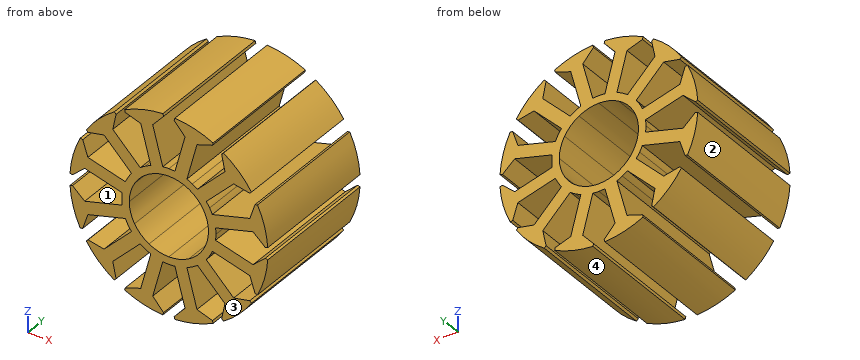
```python
from build123d import *

# Parameters (mm, degrees)
BOSS_EXTRUDE1_DEPTH = 27


with BuildPart() as part:
    # Sketch1 → Boss-Extrude1 (new body)
    with BuildSketch(Plane(origin=(0, 0, 0), x_dir=(1, 0, 0), z_dir=(0, 1, 0))):
        with BuildLine():
            Line((1.229996254, 9.420037644), (3.261041046, 17))
            Line((3.261041046, 17), (1.075459685, 19.463398226))
            Line((1.075459685, 19.463398226), (1.209434281, 19.963398226))
            ThreePointArc((1.209434281, 19.963398226), (5.176380902, 19.318516526), (8.934298302, 17.89352715))
            Line((8.934298302, 17.89352715), (8.800323705, 17.39352715))
            Line((8.800323705, 17.39352715), (5.675855612, 16.352952387))
            Line((5.675855612, 16.352952387), (3.64481082, 8.772990031))
            ThreePointArc((3.64481082, 8.772990031), (4.206265872, 8.5180589), (4.75, 8.227241336))
            ThreePointArc((4.75, 8.227241336), (5.273722462, 7.90176255), (5.775226824, 7.542993777))
            Line((5.775226824, 7.542993777), (11.324144388, 13.091911341))
            Line((11.324144388, 13.091911341), (10.66307452, 16.318067465))
            Line((10.66307452, 16.318067465), (11.029099924, 16.684092869))
            ThreePointArc((11.029099924, 16.684092869), (14.142135624, 14.142135624), (16.684092869, 11.029099924))
            Line((16.684092869, 11.029099924), (16.318067465, 10.66307452))
            Line((16.318067465, 10.66307452), (13.091911341, 11.324144388))
            Line((13.091911341, 11.324144388), (7.542993777, 5.775226824))
            ThreePointArc((7.542993777, 5.775226824), (7.90176255, 5.273722462), (8.227241336, 4.75))
            ThreePointArc((8.227241336, 4.75), (8.5180589, 4.206265872), (8.772990031, 3.64481082))
            Line((8.772990031, 3.64481082), (16.352952387, 5.675855612))
            Line((16.352952387, 5.675855612), (17.39352715, 8.800323705))
            Line((17.39352715, 8.800323705), (17.89352715, 8.934298302))
            ThreePointArc((17.89352715, 8.934298302), (19.318516526, 5.176380902), (19.963398226, 1.209434281))
            Line((19.963398226, 1.209434281), (19.463398226, 1.075459685))
            Line((19.463398226, 1.075459685), (17, 3.261041046))
            Line((17, 3.261041046), (9.420037644, 1.229996254))
            ThreePointArc((9.420037644, 1.229996254), (9.479988334, 0.61629635), (9.5, 0))
            ThreePointArc((9.5, 0), (9.479988334, -0.61629635), (9.420037644, -1.229996254))
            Line((9.420037644, -1.229996254), (17, -3.261041046))
            Line((17, -3.261041046), (19.463398226, -1.075459685))
            Line((19.463398226, -1.075459685), (19.963398226, -1.209434281))
            ThreePointArc((19.963398226, -1.209434281), (19.318516526, -5.176380902), (17.89352715, -8.934298302))
            Line((17.89352715, -8.934298302), (17.39352715, -8.800323705))
            Line((17.39352715, -8.800323705), (16.352952387, -5.675855612))
            Line((16.352952387, -5.675855612), (8.772990031, -3.64481082))
            ThreePointArc((8.772990031, -3.64481082), (8.5180589, -4.206265872), (8.227241336, -4.75))
            ThreePointArc((8.227241336, -4.75), (7.90176255, -5.273722462), (7.542993777, -5.775226824))
            Line((7.542993777, -5.775226824), (13.091911341, -11.324144388))
            Line((13.091911341, -11.324144388), (16.318067465, -10.66307452))
            Line((16.318067465, -10.66307452), (16.684092869, -11.029099924))
            ThreePointArc((16.684092869, -11.029099924), (14.142135624, -14.142135624), (11.029099924, -16.684092869))
            Line((11.029099924, -16.684092869), (10.66307452, -16.318067465))
            Line((10.66307452, -16.318067465), (11.324144388, -13.091911341))
            Line((11.324144388, -13.091911341), (5.775226824, -7.542993777))
            ThreePointArc((5.775226824, -7.542993777), (5.273722462, -7.90176255), (4.75, -8.227241336))
            ThreePointArc((4.75, -8.227241336), (4.206265872, -8.5180589), (3.64481082, -8.772990031))
            Line((3.64481082, -8.772990031), (5.675855612, -16.352952387))
            Line((5.675855612, -16.352952387), (8.800323705, -17.39352715))
            Line((8.800323705, -17.39352715), (8.934298302, -17.89352715))
            ThreePointArc((8.934298302, -17.89352715), (5.176380902, -19.318516526), (1.209434281, -19.963398226))
            Line((1.209434281, -19.963398226), (1.075459685, -19.463398226))
            Line((1.075459685, -19.463398226), (3.261041046, -17))
            Line((3.261041046, -17), (1.229996254, -9.420037644))
            ThreePointArc((1.229996254, -9.420037644), (0.61629635, -9.479988334), (0, -9.5))
            ThreePointArc((0, -9.5), (-0.61629635, -9.479988334), (-1.229996254, -9.420037644))
            Line((-1.229996254, -9.420037644), (-3.261041046, -17))
            Line((-3.261041046, -17), (-1.075459685, -19.463398226))
            Line((-1.075459685, -19.463398226), (-1.209434281, -19.963398226))
            ThreePointArc((-1.209434281, -19.963398226), (-5.176380902, -19.318516526), (-8.934298302, -17.89352715))
            Line((-8.934298302, -17.89352715), (-8.800323705, -17.39352715))
            Line((-8.800323705, -17.39352715), (-5.675855612, -16.352952387))
            Line((-5.675855612, -16.352952387), (-3.64481082, -8.772990031))
            ThreePointArc((-3.64481082, -8.772990031), (-4.206265872, -8.5180589), (-4.75, -8.227241336))
            ThreePointArc((-4.75, -8.227241336), (-5.273722462, -7.90176255), (-5.775226824, -7.542993777))
            Line((-5.775226824, -7.542993777), (-11.324144388, -13.091911341))
            Line((-11.324144388, -13.091911341), (-10.66307452, -16.318067465))
            Line((-10.66307452, -16.318067465), (-11.029099924, -16.684092869))
            ThreePointArc((-11.029099924, -16.684092869), (-14.142135624, -14.142135624), (-16.684092869, -11.029099924))
            Line((-16.684092869, -11.029099924), (-16.318067465, -10.66307452))
            Line((-16.318067465, -10.66307452), (-13.091911341, -11.324144388))
            Line((-13.091911341, -11.324144388), (-7.542993777, -5.775226824))
            ThreePointArc((-7.542993777, -5.775226824), (-7.90176255, -5.273722462), (-8.227241336, -4.75))
            ThreePointArc((-8.227241336, -4.75), (-8.5180589, -4.206265872), (-8.772990031, -3.64481082))
            Line((-8.772990031, -3.64481082), (-16.352952387, -5.675855612))
            Line((-16.352952387, -5.675855612), (-17.39352715, -8.800323705))
            Line((-17.39352715, -8.800323705), (-17.89352715, -8.934298302))
            ThreePointArc((-17.89352715, -8.934298302), (-19.318516526, -5.176380902), (-19.963398226, -1.209434281))
            Line((-19.963398226, -1.209434281), (-19.463398226, -1.075459685))
            Line((-19.463398226, -1.075459685), (-17, -3.261041046))
            Line((-17, -3.261041046), (-9.420037644, -1.229996254))
            ThreePointArc((-9.420037644, -1.229996254), (-9.479988334, -0.61629635), (-9.5, 0))
            ThreePointArc((-9.5, 0), (-9.479988334, 0.61629635), (-9.420037644, 1.229996254))
            Line((-9.420037644, 1.229996254), (-17, 3.261041046))
            Line((-17, 3.261041046), (-19.463398226, 1.075459685))
            Line((-19.463398226, 1.075459685), (-19.963398226, 1.209434281))
            ThreePointArc((-19.963398226, 1.209434281), (-19.318516526, 5.176380902), (-17.89352715, 8.934298302))
            Line((-17.89352715, 8.934298302), (-17.39352715, 8.800323705))
            Line((-17.39352715, 8.800323705), (-16.352952387, 5.675855612))
            Line((-16.352952387, 5.675855612), (-8.772990031, 3.64481082))
            ThreePointArc((-8.772990031, 3.64481082), (-8.5180589, 4.206265872), (-8.227241336, 4.75))
            ThreePointArc((-8.227241336, 4.75), (-7.90176255, 5.273722462), (-7.542993777, 5.775226824))
            Line((-7.542993777, 5.775226824), (-13.091911341, 11.324144388))
            Line((-13.091911341, 11.324144388), (-16.318067465, 10.66307452))
            Line((-16.318067465, 10.66307452), (-16.684092869, 11.029099924))
            ThreePointArc((-16.684092869, 11.029099924), (-14.142135624, 14.142135624), (-11.029099924, 16.684092869))
            Line((-11.029099924, 16.684092869), (-10.66307452, 16.318067465))
            Line((-10.66307452, 16.318067465), (-11.324144388, 13.091911341))
            Line((-11.324144388, 13.091911341), (-5.775226824, 7.542993777))
            ThreePointArc((-5.775226824, 7.542993777), (-5.273722462, 7.90176255), (-4.75, 8.227241336))
            ThreePointArc((-4.75, 8.227241336), (-4.206265872, 8.5180589), (-3.64481082, 8.772990031))
            Line((-3.64481082, 8.772990031), (-5.675855612, 16.352952387))
            Line((-5.675855612, 16.352952387), (-8.800323705, 17.39352715))
            Line((-8.800323705, 17.39352715), (-8.934298302, 17.89352715))
            ThreePointArc((-8.934298302, 17.89352715), (-5.176380902, 19.318516526), (-1.209434281, 19.963398226))
            Line((-1.209434281, 19.963398226), (-1.075459685, 19.463398226))
            Line((-1.075459685, 19.463398226), (-3.261041046, 17))
            Line((-3.261041046, 17), (-1.229996254, 9.420037644))
            ThreePointArc((-1.229996254, 9.420037644), (-0.61629635, 9.479988334), (0, 9.5))
            ThreePointArc((0, 9.5), (0.61629635, 9.479988334), (1.229996254, 9.420037644))
        make_face()
        with BuildLine():
            ThreePointArc((4, 6.92820323), (2.070552361, 7.72740661), (0, 8))
            ThreePointArc((0, 8), (-2.070552361, 7.72740661), (-4, 6.92820323))
            ThreePointArc((-4, 6.92820323), (-5.656854249, 5.656854249), (-6.92820323, 4))
            ThreePointArc((-6.92820323, 4), (-7.72740661, 2.070552361), (-8, 0))
            ThreePointArc((-8, 0), (-7.72740661, -2.070552361), (-6.92820323, -4))
            ThreePointArc((-6.92820323, -4), (-5.656854249, -5.656854249), (-4, -6.92820323))
            ThreePointArc((-4, -6.92820323), (-2.070552361, -7.72740661), (0, -8))
            ThreePointArc((0, -8), (2.070552361, -7.72740661), (4, -6.92820323))
            ThreePointArc((4, -6.92820323), (5.656854249, -5.656854249), (6.92820323, -4))
            ThreePointArc((6.92820323, -4), (7.72740661, -2.070552361), (8, 0))
            ThreePointArc((8, 0), (7.72740661, 2.070552361), (6.92820323, 4))
            ThreePointArc((6.92820323, 4), (5.656854249, 5.656854249), (4, 6.92820323))
        make_face(mode=Mode.SUBTRACT)
    extrude(amount=BOSS_EXTRUDE1_DEPTH)


solid = part.part
```
For this review, take the finished solid that the model builds, in its own axes (mm). Face numbers are marked on the shaded views. Give positions to 0.01 mm unless a question says otherwise; leave off trailing zeros. Write each loop counter-clockwise with the first axis right and the second up, starting at its lowest first coordinate (ties: lowest second). Pieces come first, ordered by that corner, then holes.
Item 1: Insertion check: P1, Ø8, axis at x = 7, z = 15, coming from the -Y side; P2, Ø12, axis at x = 7.5, y = 24, coming from the -Z side; P3, Ø5, axis at x = -6.5, y = 18.5, coming from the +Z side; P4, Ø8, axis at y = 19, z = -12.5, coming from the +X side. Each pin has a flat end and moves straight along its axis. Give the tip position at first contact, or say it passes through.
Item 2: Wall thickness on probe 1 along X at (y, z) = (1.25, 14); probe 2 along Z at (x, y) = (14.5, 9.5); probe 3 along Z at (x, y) = (-9, 23.5): over which ranges is each line inside the solid? List them lowest first.
Item 3: Take a section at A-A (z = -15). Give the boundary of the cut face in (x, y), and give its area (3 significant figures).
Item 4: The part is to be moulded in two halves that separate along X. For the marked faces 1, 2, 3 and 4, say which applies: +X half, -X half, draft (parallel to the pull), parting line (faces both ways), or undercut.
Established:
1. P1: stops at y = 0
1. P2: stops at z = -19.94
1. P3: stops at z = 19.6
1. P4: stops at x = 18.1
2. probe 1: x = -14.28 to -11.14, -5.05 to -2.46, 2.46 to 5.05, 11.14 to 14.28
2. probe 2: z = -13.77 to -11.04, -5.18 to -2.59, 2.59 to 5.18, 11.04 to 13.77
2. probe 3: z = -10.77 to -7.23, -3.71 to 3.71, 7.23 to 10.77
3. outline: (-13.23, 0) - (-10.93, 0) - (-10.93, 27) - (-13.23, 27) - close; (-5.31, 0) - (-2.73, 0) - (-2.73, 27) - (-5.31, 27) - close; (2.73, 0) - (5.31, 0) - (5.31, 27) - (2.73, 27) - close; (10.93, 0) - (13.23, 0) - (13.23, 27) - (10.93, 27) - close
3. area: 264 mm2
4. face 1: undercut
4. face 2: -X half
4. face 3: draft
4. face 4: +X half
